```python
from build123d import *

# Parameters (mm, degrees)
F0_W     = 32.8638516366
F0_H     = 19.1183499992
F1_DEPTH = 30
F2_DEPTH = 30
F3_DEPTH = 3
F4_DEPTH = 10.5


with BuildPart() as f1:
    # F0 (on Top) → F1 (new body)
    with BuildSketch(Plane.XY):
        Polygon((33.5817799435, 0), (33.5817799435, 30), (-33.5817799435, 30), (-33.5817799435, 0), (-16.4319258183, 0), (-16.4319258183, 19.1183499992), (16.4319258183, 19.1183499992), (16.4319258183, 0), align=None)
        with Locations((0, 9.5591749996)):
            Rectangle(F0_W, F0_H)
    extrude(amount=F1_DEPTH)

    # F0 (on Top) → F2 (join)
    with BuildSketch(Plane.XY):
        with BuildLine():
            Line((16.4319258183, -13.1183499992), (16.4319258183, 0))
            Line((16.4319258183, 0), (-16.4319258183, 0))
            Line((-16.4319258183, 0), (-16.4319258183, -13.1183499992))
            ThreePointArc((-16.4319258183, -13.1183499992), (-12.1892851312, -14.8757093121), (-10.4319258183, -19.1183499992))
            Line((-10.4319258183, -19.1183499992), (10.4319258183, -19.1183499992))
            ThreePointArc((10.4319258183, -19.1183499992), (12.1892851312, -14.8757093121), (16.4319258183, -13.1183499992))
        make_face()
        with BuildLine():
            Line((33.5817799435, -30), (33.5817799435, 0))
            Line((33.5817799435, 0), (16.4319258183, 0))
            Line((16.4319258183, 0), (16.4319258183, -13.1183499992))
            ThreePointArc((16.4319258183, -13.1183499992), (20.6745665054, -14.8757093121), (22.4319258183, -19.1183499992))
            ThreePointArc((22.4319258183, -19.1183499992), (16.4319258183, -25.1183499992), (10.4319258183, -19.1183499992))
            Line((10.4319258183, -19.1183499992), (-10.4319258183, -19.1183499992))
            ThreePointArc((-10.4319258183, -19.1183499992), (-20.6745665054, -23.3609906863), (-16.4319258183, -13.1183499992))
            Line((-16.4319258183, -13.1183499992), (-16.4319258183, 0))
            Line((-16.4319258183, 0), (-33.5817799435, 0))
            Line((-33.5817799435, 0), (-33.5817799435, -30))
            Line((-33.5817799435, -30), (33.5817799435, -30))
        make_face()
    extrude(amount=F2_DEPTH)

    # F0 (on Top) → F3 (join)
    with BuildSketch(Plane.XY):
        with BuildLine():
            Line((-16.4319258183, -17.1183499992), (-16.4319258183, -13.1183499992))
            ThreePointArc((-16.4319258183, -13.1183499992), (-20.6745665054, -23.3609906863), (-10.4319258183, -19.1183499992))
            Line((-10.4319258183, -19.1183499992), (-14.4319258183, -19.1183499992))
            ThreePointArc((-14.4319258183, -19.1183499992), (-17.8461393807, -20.5325635616), (-16.4319258183, -17.1183499992))
        make_face()
        with BuildLine():
            ThreePointArc((-10.4319258183, -19.1183499992), (-12.1892851312, -14.8757093121), (-16.4319258183, -13.1183499992))
            Line((-16.4319258183, -13.1183499992), (-16.4319258183, -17.1183499992))
            ThreePointArc((-16.4319258183, -17.1183499992), (-15.017712256, -17.7041364368), (-14.4319258183, -19.1183499992))
            Line((-14.4319258183, -19.1183499992), (-10.4319258183, -19.1183499992))
        make_face()
        with BuildLine():
            Line((16.4319258183, -17.1183499992), (16.4319258183, -13.1183499992))
            ThreePointArc((16.4319258183, -13.1183499992), (12.1892851312, -14.8757093121), (10.4319258183, -19.1183499992))
            Line((10.4319258183, -19.1183499992), (14.4319258183, -19.1183499992))
            ThreePointArc((14.4319258183, -19.1183499992), (15.017712256, -17.7041364368), (16.4319258183, -17.1183499992))
        make_face()
        with BuildLine():
            ThreePointArc((22.4319258183, -19.1183499992), (20.6745665054, -14.8757093121), (16.4319258183, -13.1183499992))
            Line((16.4319258183, -13.1183499992), (16.4319258183, -17.1183499992))
            ThreePointArc((16.4319258183, -17.1183499992), (17.8461393807, -17.7041364368), (18.4319258183, -19.1183499992))
            ThreePointArc((18.4319258183, -19.1183499992), (16.4319258183, -21.1183499992), (14.4319258183, -19.1183499992))
            Line((14.4319258183, -19.1183499992), (10.4319258183, -19.1183499992))
            ThreePointArc((10.4319258183, -19.1183499992), (16.4319258183, -25.1183499992), (22.4319258183, -19.1183499992))
        make_face()
    extrude(amount=F3_DEPTH)

    # F0 (on Top) → F4 (cut)
    with BuildSketch(Plane.XY):
        Polygon((33.5817799435, 0), (33.5817799435, 30), (-33.5817799435, 30), (-33.5817799435, 0), (-16.4319258183, 0), (-16.4319258183, 19.1183499992), (16.4319258183, 19.1183499992), (16.4319258183, 0), align=None)
        with Locations((0, 9.5591749996)):
            Rectangle(F0_W, F0_H)
    extrude(amount=F4_DEPTH, mode=Mode.SUBTRACT)


solid = f1.part
```
For this review, take the finished solid that the model builds, in its own axes (mm). A direction names the side the tool comes from. Round coordinates to 2 decimals unless told otherwise and drop trailing zeros. Write each loop counter-clockwise with the first axis right and the second up, starting at its lowest first coordinate (ties: lowest second). Pieces come first, ordered by that corner, then holes. Notation, with made-up numbers: (63.25, -22.5) - (119.25, -22.5) arc R26 cw to (119.25, 15.5) - close; hole circle Ø6 at (-22.5, 49.25). An arc over 180 degrees is marked (long way). Use CSV: the item, a comma, the result in double quotes.
1) Add section C-C on x = -17.5. Write out the cut boundary in (y, z), and give its area (3 significant figures).
Conclusion:
outline,"(-30, 0) - (-20.81, 0) - (-20.81, 3) - (-25.02, 3) - (-25.02, 30) - (-30, 30) - close; (-17.43, 0) - (0, 0) - (0, 10.5) - (30, 10.5) - (30, 30) - (-13.21, 30) - (-13.21, 3) - (-17.43, 3) - close"
area,"1,160 mm^2"
2) Add section B-B on x = -29. Write out the cut boundary in (y, z).
Conclusion:
outline,"(-30, 0) - (0, 0) - (0, 10.5) - (30, 10.5) - (30, 30) - (-30, 30) - close"
3) The part is to be moulded in two halves that separate along Y. For faces 1 (the flat face through (-14, -19, 3)), 2 (the flat face through (16, -22, 3)), 3 (the flat face through (0, -30, 15)), 4 (the flat face through (-33.582, 0, 18)), say which applies: pulls with the +Y half, pulls with the -Y half, needs draft (parallel to the pull), parting line crosses it, or undercut.
Conclusion:
face 1,"undercut"
face 2,"undercut"
face 3,"pulls with the -Y half"
face 4,"needs draft"
4) Clearance check with a flat-ended pin moving along its axis: pin 1 Ø15 at (x, y) = (-15, 21.5) entering from -Z. State where the tip first meets the part, or that it passes through.
Conclusion:
pin 1,"stops at z = 10.5"
5) Add section D-D on y = 25. Write out the cut boundary in (x, z).
Conclusion:
outline,"(-33.58, 10.5) - (33.58, 10.5) - (33.58, 30) - (-33.58, 30) - close"
6) Wall thickness on line 1 along Z through (x, y) = (11.5, 22); line 2 along Y through (x, z) = (-16.5, 25.25); line 3 along Y through (x, z) = (-21, 7.25): over which ranges is each line inside the solid? List them lowest first. Write a range as from..to.
Conclusion:
line 1,"z = 10.5..30"
line 2,"y = -30..-25.12, -13.12..30"
line 3,"y = -30..-23.01, -15.23..0"
7) Add section A-A on z = 6.25. Write out the cut boundary in (x, y), and give its area (3 significant figures).
Conclusion:
outline,"(-33.58, -30) - (33.58, -30) - (33.58, 0) - (-33.58, 0) - close; hole circle Ø12 at (-16.43, -19.12); hole circle Ø12 at (16.43, -19.12)"
area,"1,790 mm^2"
8) For faces 5 (the flat face through (0, 0, 5)), 6 (the flat face through (0, 30, 20)), list the 3-axis set-ups (+Z, -Z, +X, -X, +Y, -Y) from which the entire face can be reached by the end or side of a thin tool; tool diameter is ignored.
Conclusion:
face 5,"-Z, +X, -X, +Y"
face 6,"+Z, -Z, +X, -X, +Y"
